Read the model definition and answer for the solid it produces. Units are mm, in the model's axes. A direction names the side the tool comes from. Coordinates: 2 decimals unless noted, no trailing zeros. Write each loop counter-clockwise with the first axis right and the second up, starting at its lowest first coordinate (ties: lowest second). Pieces come first, ordered by that corner, then holes. Notation, with made-up numbers: (-4.75, -24.75) - (42.25, -24.75) arc R32 cw to (42.25, 10.25) - close; hole circle Ø7 at (-1.75, 46.25). An arc over 180 degrees is marked (long way). Return JSON: item names as keys, results as strings.
Autodesk Inventor part; units mm, degrees
ref_plane "Arbeitsebene1" through (0, 0, 0) normal (-1, 0, 0) x (0, -1, 0)
ref_plane "Arbeitsebene2" through (0, 0, 2.2393) normal (0, -1, 0) x (-1, 0, 0)
ref_plane "YZ Plane" through (0, 0, 0) normal (1, 0, 0) x (0, 1, 0)
sketch "Skizze1" plane through (0, 0, 0) normal (0, 0, 1) x (1, 0, 0)
  circle A0 centre (0, 0) radius 2.5
  line L0 (0, 2.5) -> (0, -2.5)
  dimension "d0" = 5
revolve "Umdrehung1" add sketch "Skizze1" angle 360 about axis through (0, 2.5, 0) along (0, -1, 0) picked at (0.5196, 0.6515) contours A0 L0
ref_plane "Arbeitsebene1" through (0, 0, 0) normal (-1, 0, 0) x (0, -1, 0)
sketch "Skizze2" plane through (0, 0, 0) normal (-1, 0, 0) x (0, -1, 0)
  circle A0 centre (0, 0) radius 2.5
  line L0 (1.8885, 2.6999) -> (-1.1115, 2.6999)
  line L1 (-1.1115, 2.6999) -> (-1.1115, 2.2393)
  line L2 (-1.1115, 2.2393) -> (1.8885, 2.2393)
  line L3 (1.8885, 2.2393) -> (1.8885, 2.6999)
  line L4 (1.8885, 2.6999) -> (-1.1115, 2.2393) construction
  line L5 (-1.1115, 2.6999) -> (1.8885, 2.2393) construction
  point P0 (0.3885, 2.4696)
  dimension "d2" = 3
extrude "Extrusion1" cut sketch "Skizze2" along normal mid plane 10 contours L1 L0 L3 L2 A0 | A0 L2 picked at (0.1903, 2.3042)
ref_plane "Arbeitsebene2" through (0, 0, 2.2393) normal (0, -1, 0) x (-1, 0, 0)
sketch "Skizze3" plane through (0, 0, 2.2393) normal (0, -1, 0) x (-1, 0, 0)
  arc A0 (1.1115, 0) -> (-1.1115, 0) centre (0, 2.2393) ccw
  line L0 (-2.6999, 0.3508) -> (-2.2393, 0.3508)
  line L1 (-2.2393, 0.3508) -> (-2.2393, 3.3508)
  line L2 (-2.2393, 3.3508) -> (-2.6999, 3.3508)
  line L3 (-2.6999, 3.3508) -> (-2.6999, 0.3508)
  line L4 (-2.6999, 0.3508) -> (-2.2393, 3.3508) construction
  line L5 (-2.2393, 0.3508) -> (-2.6999, 3.3508) construction
  point P0 (-2.4696, 1.8508)
  dimension "d5" = 3
extrude "Extrusion2" cut sketch "Skizze3" along normal mid plane 10
sketch "Skizze4" plane through (0, 0, 0) normal (-1, 0, 0) x (0, -1, 0)
  arc A0 (-1.1115, 2.2393) -> (1.1115, 2.2393) centre (0, 0) ccw
  line L0 (-2.6999, 1.8885) -> (-2.2393, 1.8885)
  line L1 (-2.2393, 1.8885) -> (-2.2393, -1.1115)
  line L2 (-2.2393, -1.1115) -> (-2.6999, -1.1115)
  line L3 (-2.6999, -1.1115) -> (-2.6999, 1.8885)
  line L4 (-2.6999, 1.8885) -> (-2.2393, -1.1115) construction
  line L5 (-2.2393, 1.8885) -> (-2.6999, -1.1115) construction
  point P0 (-2.4696, 0.3885)
  dimension "d8" = 3
extrude "Extrusion3" cut sketch "Skizze4" along normal mid plane 10
sketch "Skizze5" plane through (2.2393, 0, 0) normal (1, 0, 0) x (0, 0, -1)
  circle A0 centre (0, 0) radius 1.1115
  circle A1 centre (0, 0) radius 0.5
  dimension "d26" = 1
sketch "Skizze6" plane through (0, 0, 2.2393) normal (0, 0, 1) x (1, 0, 0)
  circle A0 centre (0, 0) radius 1.1115
  circle A1 centre (0, 0) radius 0.5
  dimension "d27" = 1
sketch "Skizze7" plane through (0, 2.2393, 0) normal (0, 1, 0) x (1, 0, 0)
  circle A0 centre (0, 0) radius 1.1115
  circle A1 centre (0, 0) radius 0.5
  dimension "d28" = 1
extrude "Extrusion7" cut sketch "Skizze6" against normal blind 1.5 contours A1
extrude "Extrusion8" cut sketch "Skizze5" against normal blind 1.5 contours A1
extrude "Extrusion9" cut sketch "Skizze7" against normal blind 1.5 contours A1
properties part number "xyz_Axis_with_ball_Ball"
(1) A cutting plane is placed at D-D (y = -0.95). Determine the outline of the cut face in (x, z), and give its area (3 significant figures).
Answer:
{"outline": "(-0.58, 2.24) arc R2.31 ccw (long way) to (2.24, -0.58) - (2.24, 0.58) arc R2.31 ccw to (0.58, 2.24) - close", "area": "16.7 mm²"}
(2) Flat-ended cylindrical pins translate along their axes: P1, Ø0.8, axis at y = 0, z = 0, coming from the +X side; P2, Ø1, axis at x = 0.5, y = -1, coming from the -Z side; P3, Ø2, axis at y = 1, z = 0.5, coming from the -X side; P4, Ø2, axis at x = 0, y = 0, coming from the +Z side. Find the tip coordinate at first contact, or state that the pin passes through.
Answer:
{"P1": "x = 0.74", "P2": "z = -2.42", "P3": "x = -2.5", "P4": "z = 2.24"}
(3) Which of the six approach directions +Z, -Z, +X, -X, +Y, -Y give full straight-line access (tool end or side, diameter ignored) to faces 1 (the face through (0, 0.739, 0)), 2 (the face through (0.739, 0, 0))?
Answer:
{"face 1": "+Y", "face 2": "+X"}
(4) Straight lines are drawn through the part: line 1 (Y direction, x = 1.7, z = 0); line 2 (Z direction, x = 1, y = -0.15); line 3 (Y direction, x = 0.1, z = 1.6). For each, find the intervals that lie inside material, in ascending order. Write a range as from..to.
Answer:
{"line 1": "-1.83..-0.5, 0.5..1.83", "line 2": "-2.29..-0.48, 0.48..2.24", "line 3": "-1.92..-0.49, 0.49..1.92"}
(5) A cutting plane is placed at B-B (x = 1). Determine the outline of the cut face in (y, z).
Answer:
{"outline": "(-0.49, 2.24) arc R2.29 ccw (long way) to (2.24, -0.49) - (2.24, 0.49) arc R2.29 ccw to (0.49, 2.24) - close; hole circle Ø1 at (0, 0)"}
(6) A cutting plane is placed at A-A (z = 0). Determine the outline of the cut face in (x, y).
Answer:
{"outline": "(-1.11, 2.24) arc R2.5 ccw (long way) to (2.24, -1.11) - (2.24, -0.5) - (0.74, -0.5) - (0.74, 0.5) - (2.24, 0.5) - (2.24, 1.11) arc R2.5 ccw to (1.11, 2.24) - (0.5, 2.24) - (0.5, 0.74) - (-0.5, 0.74) - (-0.5, 2.24) - close"}
(7) Determine the mould class of faces 3 (the face through (-0.108, 1.5, 0.488)), 4 (the face through (0, 0, 0.739)), 5 (the face through (-0.108, -0.488, 1.5)) for opening direction Z: +Z half, -Z half, draft (parallel to the pull), parting line (faces both ways), or undercut.
Answer:
{"face 3": "undercut", "face 4": "+Z half", "face 5": "draft"}
(8) A cutting plane is placed at C-C (x = -0.2). Determine the outline of the cut face in (y, z).
Answer:
{"outline": "(-1.09, 2.24) arc R2.49 ccw (long way) to (2.24, -1.09) - (2.24, -0.46) - (0.74, -0.46) - (0.74, 0.46) - (2.24, 0.46) - (2.24, 1.09) arc R2.49 ccw to (1.09, 2.24) - (0.46, 2.24) - (0.46, 0.74) - (-0.46, 0.74) - (-0.46, 2.24) - close"}
